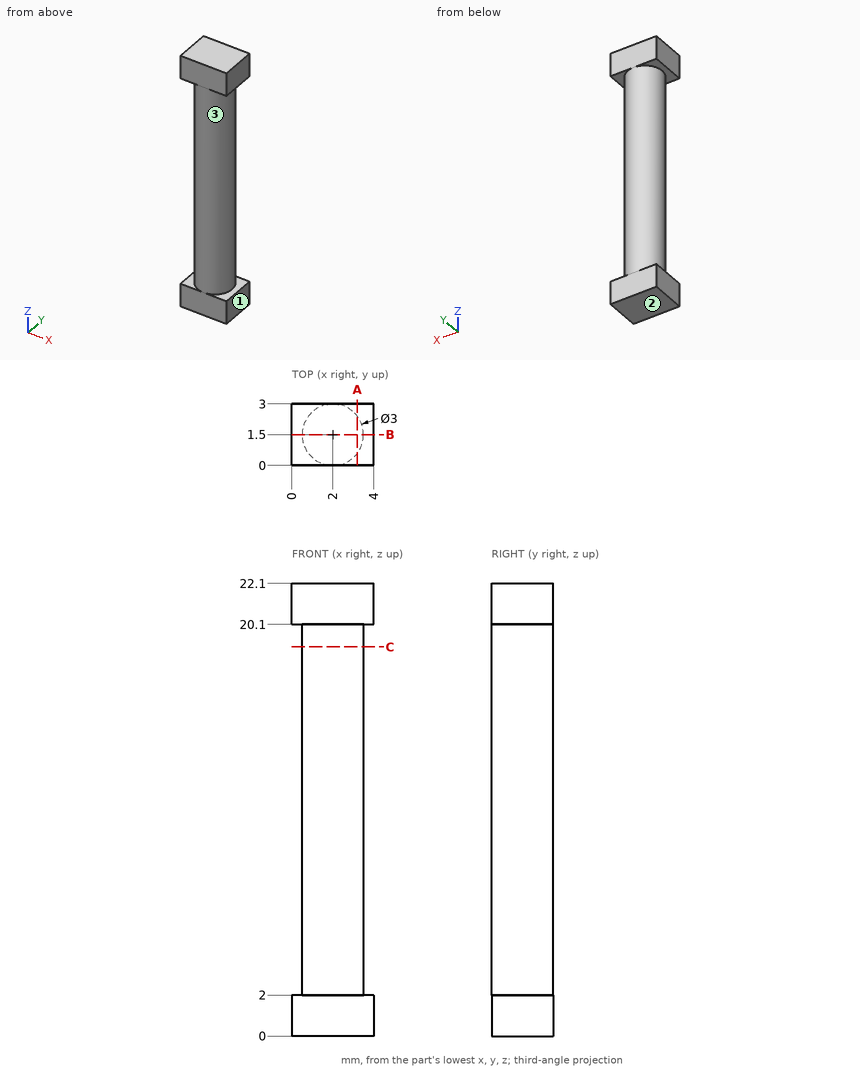
The drawing under review shows one solid part. Ordinate dimensions are in mm from its lowest x, y, z. Round coordinates to 2 decimals unless told otherwise and drop trailing zeros. Write each loop counter-clockwise with the first axis right and the second up, starting at its lowest first coordinate (ties: lowest second). Pieces come first, ordered by that corner, then holes. Notation, with made-up numbers: (-5, -8.75) - (8, -8.75) arc R25 ccw to (8, 8.25) - close; hole circle Ø1 at (71.25, 25.25). An arc over 180 degrees is marked (long way). Use a Markdown table: item, result. Add a question column.
1. We need section A-A (x = 3.2). State the section outline as (y, z) points, then the cut area to 3 significant figures.
2. We need section B-B (y = 1.5). State the section outline as (x, z) points, then the cut area to 3 significant figures.
3. Mouldability with a two-part tool opening along Z and no side actions: class the marked faces 1, 2 and 3 as +Z half, -Z half, draft (parallel to the pull), parting line (faces both ways), or undercut.
4. We need section C-C (z = 19). State the section outline as (x, y) points.
5. Wall thickness on probe 1 along Z at (x, y) = (0.2, 0.35); probe 2 along X at (y, z) = (2.5, 6.75); probe 3 along Y at (x, z) = (1.85, 16.5): over which ranges is each line inside the solid? List them lowest first.
6. Clearance check with flat-ended pins moving along their axes: pin 1 (1 mm diameter, centred on x = 1, z = 10, fed in from -Y); pin 2 (2 mm diameter, centred on x = 2.5, z = 7, fed in from +Y). State where each tip first meets the part, or that it passes through.
Output:
| question | item | result |
|---|---|---|
| 1 | outline | (0, 0) - (3, 0) - (3, 2) - (2.4, 2) - (2.4, 20.1) - (3, 20.1) - (3, 22.1) - (0, 22.1) - (0, 20.1) - (0.6, 20.1) - (0.6, 2) - (0, 2) - close |
| 1 | area | 44.6 mm2 |
| 2 | outline | (0, 0) - (4, 0) - (4, 2) - (3.5, 2) - (3.5, 20.1) - (4, 20.1) - (4, 22.1) - (0, 22.1) - (0, 20.1) - (0.5, 20.1) - (0.5, 2) - (0, 2) - close |
| 2 | area | 70.3 mm2 |
| 3 | face 1 | draft |
| 3 | face 2 | -Z half |
| 3 | face 3 | undercut |
| 4 | outline | circle Ø3 at (2, 1.5) |
| 5 | probe 1 | z = 0 to 2, 20.1 to 22.1 |
| 5 | probe 2 | x = 0.88 to 3.12 |
| 5 | probe 3 | y = 0.01 to 2.99 |
| 6 | pin 1 | stops at y = 0.09 |
| 6 | pin 2 | stops at y = 3 |
